```python
from build123d import *

# Parameters (mm, degrees)
SKETCH1_W           = 140
SKETCH1_H           = 15
BOSS_EXTRUDE1_DEPTH = 20
SKETCH2_R           = 1.8
CUT_EXTRUDE1_DEPTH  = 74.186405842
FILLET1_R           = 5
CUT_EXTRUDE2_DEPTH  = 74.186405842
LPATTERN1_COUNT     = 42
LPATTERN1_PITCH     = 7.5
FILLET2_R           = 5


with BuildPart() as part:
    # Sketch1 → Boss-Extrude1 (new body)
    with BuildSketch(Plane(origin=(0, 0, 0), x_dir=(1, 0, 0), z_dir=(0, 1, 0))):
        Rectangle(SKETCH1_W, SKETCH1_H)
    extrude(amount=BOSS_EXTRUDE1_DEPTH)

    # Sketch2 → Cut-Extrude1 (cut, through all)
    with BuildSketch(Plane(origin=(0, 20, 0), x_dir=(1, 0, 0), z_dir=(0, 1, 0))):
        with Locations(Location((-65, 2.5, 0), (0, 0, 270))):
            Circle(SKETCH2_R)
        with Locations(Location((0, 2.5, 0), (0, 0, 270))):
            Circle(SKETCH2_R)
        with Locations(Location((65, 2.5, 0), (0, 0, 270))):
            Circle(SKETCH2_R)
    extrude(amount=-CUT_EXTRUDE1_DEPTH, mode=Mode.SUBTRACT)

    # Fillet1
    fillet1_edges = [part.edges().sort_by_distance(p)[0] for p in [
        (-70, 10, -7.5),
        (70, 10, -7.5),
    ]]
    fillet(fillet1_edges, radius=FILLET1_R)

    # Sketch3 → Cut-Extrude2 (cut, through all)
    with BuildSketch(Plane(origin=(0, 20, 0), x_dir=(1, 0, 0), z_dir=(0, 1, 0))):
        with BuildLine():
            ThreePointArc((-67.834936491, -6.25), (-70, -5), (-72.165063509, -6.25))
            ThreePointArc((-72.165063509, -6.25), (-73.080127019, -7.165063509), (-74.330127019, -7.5))
            ThreePointArc((-74.330127019, -7.5), (-70, -11.830127019), (-65.669872981, -7.5))
            ThreePointArc((-65.669872981, -7.5), (-66.919872981, -7.165063509), (-67.834936491, -6.25))
        make_face()
    cut_extrude2 = extrude(amount=-CUT_EXTRUDE2_DEPTH, mode=Mode.SUBTRACT)

    # LPattern1: Cut-Extrude2 ×42
    with Locations(*[(i * LPATTERN1_PITCH, 0, 0) for i in range(1, LPATTERN1_COUNT)]):
        add(cut_extrude2, mode=Mode.SUBTRACT)

    # Fillet2
    fillet2_edges = [part.edges().sort_by_distance(p)[0] for p in [
        (-70, 10, 5),
    ]]
    fillet(fillet2_edges, radius=FILLET2_R)


solid = part.part
```
Read the model definition and answer for the solid it produces. Units are mm, in the model's axes. Give positions to 0.01 mm unless a question says otherwise; leave off trailing zeros. Put each result on its own line as item: value. Start each with the question number.
1. This flat-tipped pin is pushed along its axis until it touches: pin 1 Ø1 at (y, z) = (12.5, 3) entering from -X. Where does it stop, or does it pass through?
2. Consider line 1 along X through (y, z) = (12.5, -2.5); line 2 along Z through (x, y) = (-65, 13); line 3 along X through (y, z) = (5.25, -1.75). Determine where each line is inside the solid, lowest interval first.
3. The part is cut by section A-A, the plane y = 13.5. Give the number of separate pieces and of enclosed holes in the cut face, and give its area (3 significant figures).
4. For a pull along Z with two mould halves and no side action, classify faces 1 (the cylindrical face through (-69.58, 10.14, 3.92)), 2 (the flat face through (-1, 10, -7.5)), 3 (the flat face through (-1, 20, 0)), 4 (the cylindrical face through (-63.215, 10.14, -2.734)) as released by +Z, released by -Z, zero draft, split by the parting line, or undercut.
Final values:
1. pin 1: stops at x = -69.97
2. line 1: x = -70 to -66.8, -63.2 to -1.8, 1.8 to 63.2, 66.8 to 70
2. line 2: z = -7.5 to -4.3, -0.7 to 6.7
2. line 3: x = -70 to -66.64, -63.36 to -1.64, 1.64 to 63.36, 66.64 to 70
3. separate pieces: 1
3. enclosed holes: 3
3. area: 1,860 mm²
4. face 1: released by +Z
4. face 2: released by -Z
4. face 3: zero draft
4. face 4: undercut
